Can you work these out from the model? Positions are in its coordinate system, mm. Face numbers are marked on the shaded views. A direction names the side the tool comes from. Coordinates: 2 decimals unless noted, no trailing zeros. Order: outer loops, then holes, each group sorted by start corner. A loop starts at its lowest first (then second) coordinate and runs counter-clockwise, first axis right, second up. Notation, with made-up numbers: (-23, -39.5) -> (-8, -39.5) arc R18 cw to (-8, -23.5) -> close; hole circle Ø1 at (63, 71). An arc over 180 degrees is marked (long way). Answer as a JSON object with one key per item and string values. Group by question number.
(1) For pin 1 (6 mm diameter, centred on x = 160, y = 40, fed in from +Z), with a flat end and sliding along its axis, tell me the tip position at first contact or that it passes through.
(2) I want a section at A-A, the plane x = 125. List the corners of the cut face in (y, z) for me, plus the area to 4 significant figures.
(3) I want a section at D-D, the plane z = 41.5. List the corners of the cut face in (x, y) for me, plus the area to 4 significant figures.
(4) If we mould it in two halves opening along Y, with no side actions, what happens to the marked faces 1, 2, 3 and 4? For each: pulls with the +Y half, pulls with the -Y half, needs draft (parallel to the pull), parting line crosses it, or undercut.
(5) I need wall thicknesses on line 1 (Y direction, x = 200.5, z = 86); line 2 (X direction, y = 93, z = 130.5); line 3 (Z direction, x = 63.5, y = 81.5). Which ranges of each line are inside material? Lowest first, please.
(6) Which directions (+Z, -Z, +X, -X, +Y, -Y) give clear straight access to the entire face, cutting with the end or side of a thin tool? Please do the marked faces 5 and 6.
(7) I want a section at B-B, the plane y = 44. List the corners of the cut face in (x, z) for me, plus the area to 3 significant figures.
(8) I want a section at C-C, the plane x = 213. List the corners of the cut face in (y, z) for me, plus the area to 3 significant figures.
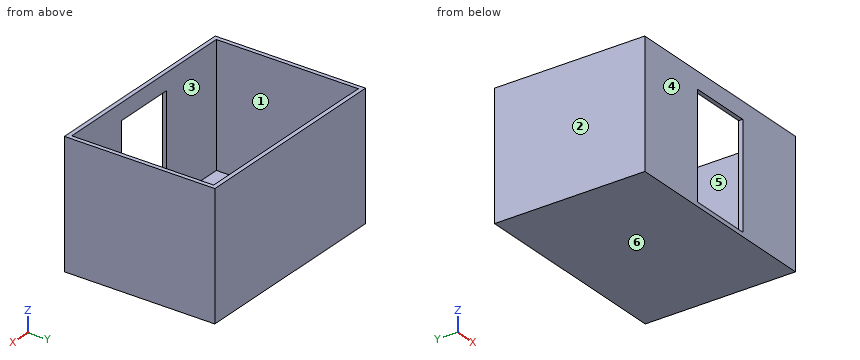
from build123d import *

# Parameters (mm, degrees)
SKETCH_W        = 250
SKETCH_H        = 180
PAD_DEPTH       = 150
SKETCH001_W     = 240
SKETCH001_H     = 170
POCKET_DEPTH    = 145
SKETCH002_W     = 75
SKETCH002_H     = 125
POCKET001_DEPTH = 5


with BuildPart() as part:
    # Sketch → Pad (new body)
    with BuildSketch(Plane.XY):
        with Locations((125, 90)):
            Rectangle(SKETCH_W, SKETCH_H)
    extrude(amount=PAD_DEPTH)

    # Sketch001 (on Face6 of Pad) → Pocket (cut)
    with BuildSketch(Plane.XY.offset(150)):
        with Locations((125, 90)):
            Rectangle(SKETCH001_W, SKETCH001_H)
    extrude(amount=-POCKET_DEPTH, mode=Mode.SUBTRACT)

    # Sketch002 (on Face6 of Pocket) → Pocket001 (cut)
    with BuildSketch(Plane.XZ):
        with Locations((125, 67.5)):
            Rectangle(SKETCH002_W, SKETCH002_H)
    extrude(amount=-POCKET001_DEPTH, mode=Mode.SUBTRACT)


solid = part.part
Computed values:
{
 "1": {"pin 1": "stops at z = 5"},
 "2": {"outline": "(0, 0) -> (180, 0) -> (180, 150) -> (175, 150) -> (175, 5) -> (0, 5) -> close; (0, 130) -> (5, 130) -> (5, 150) -> (0, 150) -> close", "area": "1,725 mm2"},
 "3": {"outline": "(0, 0) -> (87.5, 0) -> (87.5, 5) -> (5, 5) -> (5, 175) -> (245, 175) -> (245, 5) -> (162.5, 5) -> (162.5, 0) -> (250, 0) -> (250, 180) -> (0, 180) -> close", "area": "3,825 mm2"},
 "4": {"face 1": "undercut", "face 2": "needs draft", "face 3": "undercut", "face 4": "pulls with the -Y half"},
 "5": {"line 1": "y = 0 to 5, 175 to 180", "line 2": "x = 0 to 5, 245 to 250", "line 3": "z = 0 to 5"},
 "6": {"face 5": "+Z", "face 6": "-Z, +X, -X, +Y, -Y"},
 "7": {"outline": "(0, 0) -> (250, 0) -> (250, 150) -> (245, 150) -> (245, 5) -> (5, 5) -> (5, 150) -> (0, 150) -> close", "area": "2,700 mm2"},
 "8": {"outline": "(0, 0) -> (180, 0) -> (180, 150) -> (175, 150) -> (175, 5) -> (5, 5) -> (5, 150) -> (0, 150) -> close", "area": "2,350 mm2"}
}
